from build123d import *

# Parameters (mm, degrees)
CROQUIS1_W              = 53
CROQUIS1_H              = 29
SALIENTE_EXTRUIR1_DEPTH = 10.5
REDONDEO1_R             = 6
REDONDEO2_R             = 1
SALIENTE_EXTRUIR2_DEPTH = 35
CROQUIS3_W              = 3.5
CROQUIS3_H              = 6.5
SALIENTE_EXTRUIR3_DEPTH = 13.5


with BuildPart() as part:
    # Croquis1 → Saliente-Extruir1 (new body)
    with BuildSketch(Plane(origin=(0, 0, 0), x_dir=(0, 1, 0), z_dir=(0, 0, 1))):
        Rectangle(CROQUIS1_W, CROQUIS1_H)
    extrude(amount=SALIENTE_EXTRUIR1_DEPTH)

    # Redondeo1
    # the kernel refuses this fillet: 6 mm, written as the material it takes off along each edge
    with BuildSketch(Plane(origin=(29.5, -26.5, 0), x_dir=(0, 0, 1), z_dir=(-1, 0, 0))) as redondeo1_piece_1:
        with BuildLine():
            CenterArc((REDONDEO1_R, REDONDEO1_R), REDONDEO1_R, 180, 90)
            Line((0, REDONDEO1_R), (0, 0))
            Line((0, 0), (REDONDEO1_R, 0))
        make_face()
    extrude(amount=59, mode=Mode.SUBTRACT)
    with BuildSketch(Plane(origin=(29.5, -26.5, 10.5), x_dir=(0, 0, -1), z_dir=(-1, 0, 0))) as redondeo1_piece_2:
        with BuildLine():
            CenterArc((REDONDEO1_R, -REDONDEO1_R), REDONDEO1_R, 90, 90)
            Line((0, -REDONDEO1_R), (0, 0))
            Line((0, 0), (REDONDEO1_R, 0))
        make_face()
    extrude(amount=59, mode=Mode.SUBTRACT)

    # Redondeo2
    redondeo2_edges = [part.edges().sort_by_distance(p)[0] for p in [
        (14.5, 3, 0),
        (14.5, 3, 10.5),
        (14.5, -24.468626967, 9),
        (14.5, -24.468626967, 1.5),
        (-14.5, -24.468626967, 9),
        (-14.5, -24.468626967, 1.5),
        (0, 26.5, 10.5),
        (-14.5, 3, 0),
        (0, 26.5, 0),
        (14.5, 26.5, 5.25),
        (-14.5, 26.5, 5.25),
        (-14.5, 3, 10.5),
    ]]
    fillet(redondeo2_edges, radius=REDONDEO2_R)

    # Croquis2 → Saliente-Extruir2 (add)
    with BuildSketch(Plane(origin=(-14.5, 0, 0), x_dir=(0, -1, 0), z_dir=(-1, 0, 0))):
        with BuildLine():
            Line((24.543429983, 7), (24.743429983, 7))
            ThreePointArc((24.743429983, 7), (25.23840473, 6.794974747), (25.443429983, 6.3))
            Line((25.443429983, 6.3), (25.443429983, 4.2))
            ThreePointArc((25.443429983, 4.2), (25.23840473, 3.705025253), (24.743429983, 3.5))
            Line((24.743429983, 3.5), (24.543429983, 3.5))
            ThreePointArc((24.543429983, 3.5), (24.048455236, 3.705025253), (23.843429983, 4.2))
            Line((23.843429983, 4.2), (23.843429983, 6.3))
            ThreePointArc((23.843429983, 6.3), (24.048455236, 6.794974747), (24.543429983, 7))
        make_face()
    extrude(amount=SALIENTE_EXTRUIR2_DEPTH)

    # Croquis3 → Saliente-Extruir3 (add)
    with BuildSketch(Plane(origin=(-49.5, 0, 0), x_dir=(0, -1, 0), z_dir=(-1, 0, 0))):
        with Locations((24.643429983, 5.25)):
            Rectangle(CROQUIS3_W, CROQUIS3_H)
    extrude(amount=SALIENTE_EXTRUIR3_DEPTH)


solid = part.part
Read the model definition and answer for the solid it produces. Units are mm, in the model's axes. A direction names the side the tool comes from. Give positions to 0.01 mm unless a question says otherwise; leave off trailing zeros. Loops run counter-clockwise (first coordinate to the right, second up) from the corner with the lowest first, then second, coordinate; pieces in that order, holes last. Notation, with made-up numbers: (55, 44.25) -> (81, 44.25) arc R16 ccw to (81, 56.25) -> close; hole circle Ø4 at (50.25, -1). An arc over 180 degrees is marked (long way). Answer as CSV lines item,"result".
Item 1: Find section B-B on x = -23.5. Give the vertices of the cut face in (y, z).
Returned:
outline,"(-25.44, 4.2) arc R0.7 ccw to (-24.74, 3.5) -> (-24.54, 3.5) arc R0.7 ccw to (-23.84, 4.2) -> (-23.84, 6.3) arc R0.7 ccw to (-24.54, 7) -> (-24.74, 7) arc R0.7 ccw to (-25.44, 6.3) -> close"
Item 2: Find section C-C on x = 9.5. Give the vertices of the cut face in (y, z), plus the area to 3 significant figures.
Returned:
outline,"(-26.45, 5.25) arc R6 ccw to (-20.5, 0) -> (25.5, 0) arc R1 ccw to (26.5, 1) -> (26.5, 9.5) arc R1 ccw to (25.5, 10.5) -> (-20.5, 10.5) arc R6 ccw to start"
area,"541 mm²"
Item 3: Each of these flat-tipped pins is pushed along its axis until it touches: pin 1 (3 mm diameter, centred on x = -55.5, y = -24.5, fed in from +Z); pin 2 (1 mm diameter, centred on x = -40.5, z = 5.5, fed in from -Y); pin 3 (3 mm diameter, centred on x = -59.5, y = -25.5, fed in from -Z). Where does it stop, or does it pass through?
Returned:
pin 1,"stops at z = 8.5"
pin 2,"stops at y = -25.44"
pin 3,"stops at z = 2"
Item 4: Find section A-A on y = 15. Give the vertices of the cut face in (x, z).
Returned:
outline,"(-14.5, 1) arc R1 ccw to (-13.5, 0) -> (13.5, 0) arc R1 ccw to (14.5, 1) -> (14.5, 9.5) arc R1 ccw to (13.5, 10.5) -> (-13.5, 10.5) arc R1 ccw to (-14.5, 9.5) -> close"
Item 5: For faces 1 (the face through (-56, -25, 2)), 2 (the face through (0.189, -24.514, 8.96)), 3 (the face through (0.19, -24.42, 1.46)), 4 (the face through (-32, -23.843, 5)), 5 (the face through (-56, -22.893, 5)), determine the directions among +Z, -Z, +X, -X, +Y, -Y from which every point of the face is accessible in a straight line to the end or side of a thin tool.
Returned:
face 1,"-Z, -X, +Y, -Y"
face 2,"+Z, +X, -Y"
face 3,"-Z, +X, -Y"
face 4,"+Z, -Z, +Y"
face 5,"+Z, -Z, -X, +Y"
Item 6: Consider line 1 (X direction, y = -9.5, z = 5); line 2 (Y direction, x = -57, z = 6.75); line 3 (Y direction, x = -6, z = 2.5). Determine where each line is inside the solid, lowest interval first. Write a range as [from, to].
Returned:
line 1,"x = [-14.5, 14.5]"
line 2,"y = [-26.39, -22.89]"
line 3,"y = [-25.37, 26.5]"
Item 7: Determine the mould class of faces 6 (the face through (14.5, 0, 5)), 7 (the face through (-49.5, -23.5, 5.3)), 8 (the face through (0, 2, 0)) for opening direction X: +X half, -X half, draft (parallel to the pull), parting line (faces both ways), or undercut.
Returned:
face 6,"+X half"
face 7,"undercut"
face 8,"draft"
Item 8: Find section D-D on x = -55. Give the vertices of the cut face in (y, z), plus the area to 4 significant figures.
Returned:
outline,"(-26.39, 2) -> (-22.89, 2) -> (-22.89, 8.5) -> (-26.39, 8.5) -> close"
area,"22.75 mm²"
